Read the model definition and answer for the solid it produces. Units are mm, in the model's axes. Face numbers are marked on the shaded views. A direction names the side the tool comes from. Give positions to 0.01 mm unless a question says otherwise; leave off trailing zeros. Order: outer loops, then holes, each group sorted by start corner. A loop starts at its lowest first (then second) coordinate and runs counter-clockwise, first axis right, second up. Notation, with made-up numbers: (53.25, 21) -> (67.25, 21) arc R19 ccw to (67.25, 39) -> close; hole circle Ø3 at (-5, 12.25). An arc over 180 degrees is marked (long way). Use one line per item in the form item = value.
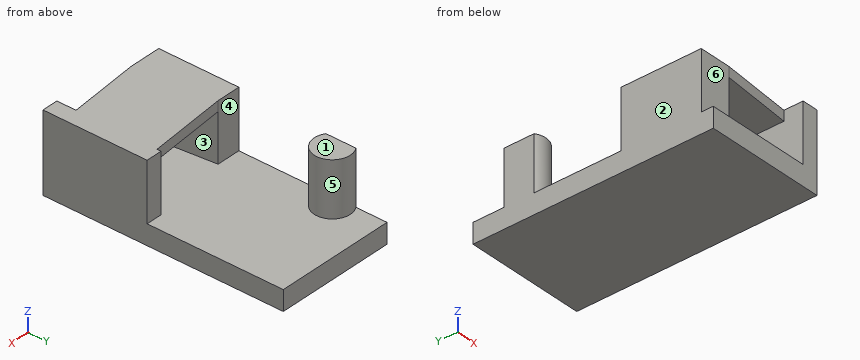
```python
from build123d import *

# Parameters (mm, degrees)
SKETCH1_W           = 60
SKETCH1_H           = 120
BOSS_EXTRUDE1_DEPTH = 10
SKETCH3_R           = 9
BOSS_EXTRUDE3_DEPTH = 27
CUT_EXTRUDE1_DEPTH  = 38
SKETCH5_W           = 16
SKETCH5_H           = 40
BOSS_EXTRUDE4_DEPTH = 29
SKETCH2_W           = 8
SKETCH2_H           = 52
BOSS_EXTRUDE5_DEPTH = 29
CUT_EXTRUDE2_DEPTH  = 29
SKETCH9_W           = 5
SKETCH9_H           = 40.199502484
BOSS_EXTRUDE6_DEPTH = 42


with BuildPart() as part:
    # Sketch1 → Boss-Extrude1 (new body)
    with BuildSketch(Plane.XY):
        with Locations((30, 60)):
            Rectangle(SKETCH1_W, SKETCH1_H)
    extrude(amount=BOSS_EXTRUDE1_DEPTH)

    # Sketch3 → Boss-Extrude3 (add)
    with BuildSketch(Plane.XY.offset(10)):
        with Locations((5, 97)):
            Circle(SKETCH3_R)
    extrude(amount=BOSS_EXTRUDE3_DEPTH)

    # Sketch4 → Cut-Extrude1 (cut, through all)
    with BuildSketch(Plane.XY.offset(37)):
        Polygon((0, 104.483314774), (0, 89.516685226), (-21.075421501, 89.516685226), (-21.075421501, 106.99834991), align=None)
    extrude(amount=-CUT_EXTRUDE1_DEPTH, mode=Mode.SUBTRACT)

    # Sketch5 → Boss-Extrude4 (add)
    with BuildSketch(Plane.XY.offset(10)):
        with Locations((8, 26)):
            Rectangle(SKETCH5_W, SKETCH5_H)
    extrude(amount=BOSS_EXTRUDE4_DEPTH)

    # Sketch2 → Boss-Extrude5 (add)
    with BuildSketch(Plane.XY.offset(10)):
        with Locations((56, 26)):
            Rectangle(SKETCH2_W, SKETCH2_H)
    extrude(amount=BOSS_EXTRUDE5_DEPTH)

    # Sketch8 → Cut-Extrude2 (cut)
    with BuildSketch(Plane.XY.offset(39)):
        Polygon((16, 46), (12, 46), (16, 6), align=None)
    extrude(amount=-CUT_EXTRUDE2_DEPTH, mode=Mode.SUBTRACT)

    # Sketch9 → Boss-Extrude6 (add)
    with BuildSketch(Plane(origin=(16.435643564, 1.643564356, 0), x_dir=(0, 0, -1), z_dir=(0.99503719, 0.099503719, 0))):
        with Locations((-36.5, 24.477914879)):
            Rectangle(SKETCH9_W, SKETCH9_H)
    extrude(amount=BOSS_EXTRUDE6_DEPTH)


solid = part.part
```
Item 1: Determine the mould class of the marked faces 1, 2 and 3 for opening direction Z: +Z half, -Z half, draft (parallel to the pull), parting line (faces both ways), or undercut.
Checks:
face_1 = +Z half
face_2 = draft
face_3 = undercut
Item 2: Which of the six approach directions +Z, -Z, +X, -X, +Y, -Y give full straight-line access (tool end or side, diameter ignored) to the marked faces 4, 5 and 6?
Checks:
face_4 = +Z, -X
face_5 = +Z
face_6 = +Z, -X, -Y
Item 3: Given pin 1 Ø15.5 at (x, y) = (8.5, 94) entering from +Z; pin 2 Ø12 at (x, z) = (9, 19.5) entering from +Y; pin 3 Ø12 at (x, z) = (45, 22) entering from -Y; pin 4 Ø5 at (x, z) = (7, 17.5) entering from -Y, each flat-ended and moving along its own axis, determine where each tip first touches the part or whether it passes through.
Checks:
pin_1 = 37
pin_2 = 106
pin_3 = through
pin_4 = 6
Item 4: The part is cut by section C-C on z = 23. Give the vertices of the cut face in (x, y).
Checks:
outline = (0, 6) -> (16, 6) -> (12, 46) -> (0, 46) -> close; (0, 89.52) arc R9 ccw (long way) to (0, 104.48) -> close; (52, 0) -> (60, 0) -> (60, 52) -> (52, 52) -> close
Item 5: The part is cut by section D-D on y = 8. Give the vertices of the cut face in (x, z).
Checks:
outline = (0, 0) -> (60, 0) -> (60, 39) -> (52, 39) -> (52, 10) -> (15.8, 10) -> (15.8, 34) -> (36, 34) -> (36, 39) -> (0, 39) -> close
Item 6: Straight lines are drawn through the part: L1, parallel to Z at x = 40.5, y = 22; L2, parallel to Z at x = 16.5, y = 56.5; L3, parallel to Y at x = 4.5, z = 24.5. For each, find the intervals that lie inside material, in ascending order. Write a range as from..to.
Checks:
L1 = 0..10, 34..39
L2 = 0..10
L3 = 6..46, 88.01..105.99
Item 7: The part is cut by section B-B on y = 36.5. Give the vertices of the cut face in (x, z).
Checks:
outline = (0, 0) -> (60, 0) -> (60, 39) -> (0, 39) -> close; hole (12.95, 10) -> (52, 10) -> (52, 34) -> (12.95, 34) -> close
Item 8: The part is cut by section A-A on x = 47.5. Give the vertices of the cut face in (y, z), and give its area (3 significant figures).
Checks:
outline = (0, 0) -> (120, 0) -> (120, 10) -> (0, 10) -> close; (9.15, 34) -> (49.55, 34) -> (49.55, 39) -> (9.15, 39) -> close
area = 1,400 mm²
